from build123d import *

# Parameters (mm, degrees)
SKETCH_1_W             = 800
SKETCH_1_H             = 400
EXTRUDE_1_DEPTH        = 20
SKETCH_2_W             = 111
SKETCH_2_H             = 41
CUT_EXTRUDE_1_DEPTH    = 2
HOLE_WIZARD_M6_2_D     = 5
HOLE_WIZARD_M6_2_DEPTH = 11
HOLE_WIZARD_M6_2_TIP   = 1.502151548
SKETCH_11_R            = 19.05
CUT_EXTRUDE_2_DEPTH    = 895.650769854
HOLE_WIZARD_M6_3_D     = 5
HOLE_WIZARD_M6_3_DEPTH = 13
HOLE_WIZARD_M6_3_TIP   = 1.502151548


with BuildPart() as part:
    # 스케치1 → 보스-돌출1 (new body)
    with BuildSketch(Plane.XY):
        with Locations((400, 200)):
            Rectangle(SKETCH_1_W, SKETCH_1_H)
    extrude(amount=EXTRUDE_1_DEPTH)

    # 스케치2 → 컷-돌출1 (cut)
    with BuildSketch(Plane.XY.offset(20)):
        with BuildLine():
            Line((64, 158), (97, 158))
            ThreePointArc((97, 158), (99.828427125, 156.828427125), (101, 154))
            Line((101, 154), (101, 86))
            ThreePointArc((101, 86), (99.828427125, 83.171572875), (97, 82))
            Line((97, 82), (64, 82))
            ThreePointArc((64, 82), (61.171572875, 83.171572875), (60, 86))
            Line((60, 86), (60, 154))
            ThreePointArc((60, 154), (61.171572875, 156.828427125), (64, 158))
        make_face()
        with BuildLine():
            Line((88, 220.5), (197, 220.5))
            ThreePointArc((197, 220.5), (197.707106781, 220.207106781), (198, 219.5))
            Line((198, 219.5), (198, 180.5))
            ThreePointArc((198, 180.5), (197.707106781, 179.792893219), (197, 179.5))
            Line((197, 179.5), (88, 179.5))
            ThreePointArc((88, 179.5), (87.292893219, 179.792893219), (87, 180.5))
            Line((87, 180.5), (87, 219.5))
            ThreePointArc((87, 219.5), (87.292893219, 220.207106781), (88, 220.5))
        make_face()
        with Locations((382.5, 200)):
            Rectangle(SKETCH_2_W, SKETCH_2_H)
        with BuildLine():
            Line((608, 220.5), (717, 220.5))
            ThreePointArc((717, 220.5), (717.707106781, 220.207106781), (718, 219.5))
            Line((718, 219.5), (718, 180.5))
            ThreePointArc((718, 180.5), (717.707106781, 179.792893219), (717, 179.5))
            Line((717, 179.5), (608, 179.5))
            ThreePointArc((608, 179.5), (607.292893219, 179.792893219), (607, 180.5))
            Line((607, 180.5), (607, 219.5))
            ThreePointArc((607, 219.5), (607.292893219, 220.207106781), (608, 220.5))
        make_face()
        with BuildLine():
            Line((701, 158), (734, 158))
            ThreePointArc((734, 158), (736.828427125, 156.828427125), (738, 154))
            Line((738, 154), (738, 86))
            ThreePointArc((738, 86), (736.828427125, 83.171572875), (734, 82))
            Line((734, 82), (701, 82))
            ThreePointArc((701, 82), (698.171572875, 83.171572875), (697, 86))
            Line((697, 86), (697, 154))
            ThreePointArc((697, 154), (698.171572875, 156.828427125), (701, 158))
        make_face()
    extrude(amount=-CUT_EXTRUDE_1_DEPTH, mode=Mode.SUBTRACT)

    # M6 나사 구멍2
    with Locations(Plane.XY.offset(18)):
        with Locations((162, 188.5), (162, 211.5), (122, 211.5), (122, 188.5), (93, 92.5), (68, 92.5), (68, 147.5), (93, 147.5), (362, 211.5), (402, 211.5), (402, 188.5), (362, 188.5), (642, 211.5), (682, 211.5), (682, 188.5), (642, 188.5), (706, 92.5), (731, 92.5), (731, 147.5), (706, 147.5)):
            Hole(HOLE_WIZARD_M6_2_D / 2, depth=HOLE_WIZARD_M6_2_DEPTH)
            with Locations((0, 0, -(HOLE_WIZARD_M6_2_DEPTH + HOLE_WIZARD_M6_2_TIP / 2))):  # 118° drill point
                Cone(0, HOLE_WIZARD_M6_2_D / 2, HOLE_WIZARD_M6_2_TIP, mode=Mode.SUBTRACT)

    # 스케치11 → 컷-돌출2 (cut, through all)
    with BuildSketch(Plane.XY.offset(20)):
        with Locations((535, 200)):
            Circle(SKETCH_11_R)
    extrude(amount=-CUT_EXTRUDE_2_DEPTH, mode=Mode.SUBTRACT)

    # M6 나사 구멍3
    with Locations(Plane(origin=(0, 0, 0), x_dir=(-1, 0, 0), z_dir=(0, 0, -1))):
        with Locations((-30, 10), (-70, 10), (-30, 50), (-70, 50), (-730, 10), (-770, 10), (-730, 50), (-770, 50), (-730, 390), (-770, 390), (-730, 350), (-770, 350), (-30, 390), (-70, 390), (-30, 350), (-70, 350)):
            Hole(HOLE_WIZARD_M6_3_D / 2, depth=HOLE_WIZARD_M6_3_DEPTH)
            with Locations((0, 0, -(HOLE_WIZARD_M6_3_DEPTH + HOLE_WIZARD_M6_3_TIP / 2))):  # 118° drill point
                Cone(0, HOLE_WIZARD_M6_3_D / 2, HOLE_WIZARD_M6_3_TIP, mode=Mode.SUBTRACT)


solid = part.part
The listing builds one solid part. Answer for the finished solid, in the listing's coordinates (mm). A direction names the side the tool comes from. Round coordinates to 2 decimals unless told otherwise and drop trailing zeros. Use a Markdown table: item, result. Add a question column.
1. A tool of negligible diameter and unlimited length cuts with its end or side. For faces 1 (the face through (663, 200, 18)), 2 (the face through (394, 247, 20)), from which of +Z, -Z, +X, -X, +Y, -Y can it reach the whole face along a straight path? Write none if from no direction.
2. Flat-ended cylindrical pins translate along their axes: P1, Ø4, axis at x = 731, y = 92.5, coming from the +Z side; P2, Ø23, axis at x = 535, y = 200, coming from the -Z side; P3, Ø4.5, axis at x = 402, y = 188.5, coming from the +Z side. Find the tip coordinate at first contact, or state that the pin passes through.
3. For a pull along X with two mould halves and no side action, classify faces 3 (the face through (718, 121, 18)), 4 (the face through (0, 197, 10)), 5 (the face through (394, 203, 0)) as +X half, -X half, draft (parallel to the pull), parting line (faces both ways), or undercut.
4. Consider line 1 (Y direction, x = 362, z = 14.75); line 2 (Y direction, x = 770, z = 4.5); line 3 (X direction, y = 147.5, z = 12.5). Determine where each line is inside the solid, lowest interval first.
Reported:
| question | item | result |
|---|---|---|
| 1 | face 1 | +Z |
| 1 | face 2 | +Z, +X, -X, +Y, -Y |
| 2 | P1 | z = 6.7 |
| 2 | P2 | through |
| 2 | P3 | z = 6.85 |
| 3 | face 3 | undercut |
| 3 | face 4 | -X half |
| 3 | face 5 | draft |
| 4 | line 1 | 0 to 186, 191 to 209, 214 to 400 |
| 4 | line 2 | 0 to 7.5, 12.5 to 47.5, 52.5 to 347.5, 352.5 to 387.5, 392.5 to 400 |
| 4 | line 3 | 0 to 65.5, 70.5 to 90.5, 95.5 to 703.5, 708.5 to 728.5, 733.5 to 800 |
